Can you work these out from the model? Positions are in its coordinate system, mm. Face numbers are marked on the shaded views. A direction names the side the tool comes from. Round coordinates to 2 decimals unless told otherwise and drop trailing zeros. Loops run counter-clockwise (first coordinate to the right, second up) from the corner with the lowest first, then second, coordinate; pieces in that order, holes last. Notation, with made-up numbers: M 82,-39 L 98,-39 A11 ccw 98,-31 Z; hole C 86.5,80 d11. An arc over 180 degrees is marked long. Return JSON: item names as keys, results as strings.
```python
from build123d import *

# Parameters (mm, degrees)
F1_DEPTH    = 5
F2_T1_DEPTH = 45
F2_T3_DEPTH = 44.9804639793


# Not quite as in the source:
# - a fillet or chamfer that OpenCascade refuses, or shapes differently, is made with other operations: its cross-section is extruded or revolved along the edge and cut away or added


with BuildPart() as f1:
    # F0 (on Front) → F1 (new body)
    with BuildSketch(Plane.XZ):
        Polygon((2.75, -8.5), (10.5, -8.5), (10.5, 8.5), (-10.5, 8.5), (-10.5, -8.5), (-2.75, -8.5), (-2.75, 0), (2.75, 0), align=None)
    extrude(amount=F1_DEPTH)

    # F2: fillet of radius 8 on 4 edges, made by hand

    # F2_s2 → F2_t1 (cut)
    with BuildSketch(Plane.XZ.offset(-20)):
        with BuildLine():
            ThreePointArc((-2.5, 8.5), (-8.1568542495, 6.1568542495), (-10.5, 0.5))
            Line((-10.5, 0.5), (-10.5, 8.5))
            Line((-10.5, 8.5), (-2.5, 8.5))
        make_face()
        with BuildLine():
            ThreePointArc((10.5, 0.5), (8.1568542495, 6.1568542495), (2.5, 8.5))
            Line((2.5, 8.5), (10.5, 8.5))
            Line((10.5, 8.5), (10.5, 0.5))
        make_face()
    extrude(amount=F2_T1_DEPTH, mode=Mode.SUBTRACT)

    # F2_s4 → F2_t3 (cut)
    with BuildSketch(Plane.XZ.offset(-19.9902319896)):
        with BuildLine():
            ThreePointArc((2.75, -8.5), (8.2445626465, -6.071671567), (10.5, -0.5039072041))
            Line((10.5, -0.5039072041), (10.5, -8.5))
            Line((10.5, -8.5), (2.75, -8.5))
        make_face()
        with BuildLine():
            ThreePointArc((-10.5, -0.5039072041), (-8.2445626465, -6.071671567), (-2.75, -8.5))
            Line((-2.75, -8.5), (-10.5, -8.5))
            Line((-10.5, -8.5), (-10.5, -0.5039072041))
        make_face()
    extrude(amount=F2_T3_DEPTH, mode=Mode.SUBTRACT)


solid = f1.part
```
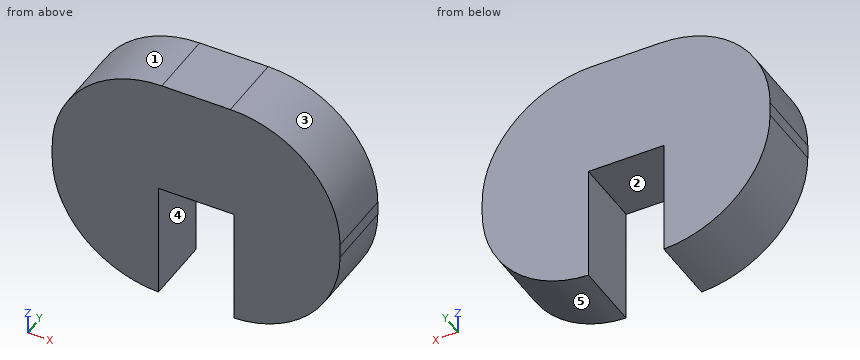
Q1. I'm going to push flat-ended pins straight in: pin 1 Ø2.5 at (y, z) = (-3, -4.5) entering from +X; pin 2 Ø2 at (x, y) = (0, -2.5) entering from -Z; pin 3 Ø1.5 at (y, z) = (-4.5, -6.5) entering from +X. Where does each tip first touch, or does it pass through?
Results:
{"pin 1": "stops at x = 10.01", "pin 2": "stops at z = 0", "pin 3": "stops at x = 8.54"}
Q2. Suppose I cut it at A-A, the plane y = -3.1. Please give me the cut outline in (x, z), plus the area to 3 significant figures.
Results:
{"outline": "M -10.5,-0.5 A8 ccw -2.75,-8.5 L -2.75,0 L 2.75,0 L 2.75,-8.5 A8 ccw 10.5,-0.5 L 10.5,0.5 A8 ccw 2.5,8.5 L -2.5,8.5 A8 ccw -10.5,0.5 Z", "area": "255 mm2"}
Q3. Suppose I cut it at B-B, the plane z = -4.75. Please give me the cut outline in (x, y), plus the area to 3 significant figures.
Results:
{"outline": "M -9.28,-5 L -2.75,-5 L -2.75,0 L -9.28,0 Z; M 2.75,-5 L 9.28,-5 L 9.28,0 L 2.75,0 Z", "area": "65.3 mm2"}
Q4. Thinking about a two-plate mould opening in X: for the marked faces 1, 2 and 3, which applies, pulls with the +X half, pulls with the -X half, needs draft (parallel to the pull), parting line crosses it, or undercut?
Results:
{"face 1": "pulls with the -X half", "face 2": "undercut", "face 3": "pulls with the +X half"}
Q5. Suppose I cut it at D-D, the plane z = -2. Please give me the cut outline in (x, y), plus the area to 3 significant figures.
Results:
{"outline": "M -10.36,-5 L -2.75,-5 L -2.75,0 L -10.36,0 Z; M 2.75,-5 L 10.36,-5 L 10.36,0 L 2.75,0 Z", "area": "76.1 mm2"}
Q6. On a 3-axis mill with a long thin cutter (end or side, diameter ignored), from which of +Z, -Z, +X, -X, +Y, -Y can I reach the whole of each face in a straight line? I mean the marked faces 4 and 5. Say none if no direction works.
Results:
{"face 4": "-Z, +Y, -Y", "face 5": "-Z, +X, +Y, -Y"}
Q7. Suppose I cut it at C-C, the plane x = 1. Please give me the cut outline in (y, z), plus the area to 3 significant figures.
Results:
{"outline": "M -5,0 L 0,0 L 0,8.5 L -5,8.5 Z", "area": "42.5 mm2"}
Q8. If I drill on line 1 along Z through (x, y) = (-2.25, -3.35); line 2 along X through (y, z) = (-1.35, -7); line 3 along X through (y, z) = (-3.1, -2), over which ranges is the centre line in solid material (lowest first)?
Results:
{"line 1": "z = 0 to 8.5", "line 2": "x = -7.17 to -2.75, 2.75 to 7.17", "line 3": "x = -10.36 to -2.75, 2.75 to 10.36"}
